```python
from build123d import *

# Parameters (mm, degrees)
SKETCH_1_R               = 6.325
EXTRUDE_1_DEPTH          = 15
SKETCH_2_W               = 20.7
SKETCH_2_H               = 20
EXTRUDE_2_DEPTH          = 5
SKETCH_3_W               = 5
SKETCH_3_H               = 20
EXTRUDE_3_DEPTH          = 10.2
SKETCH_4_R               = 1.7
CUT_EXTRUDE_1_DEPTH      = 21.932331452
CUT_EXTRUDE_1_DEPTH_BACK = 21.932331452
SKETCH_5_R               = 1.65
CUT_EXTRUDE_2_DEPTH      = 21.932331452
CUT_EXTRUDE_2_DEPTH_BACK = 21.932331452
SKETCH_6_R               = 1.75
EXTRUDE_4_DEPTH          = 5
CHAMFER_2_SIZE           = 1
CHAMFER_3_SIZE           = 1
CUT_EXTRUDE_3_DEPTH      = 33.153149146
CUT_EXTRUDE_3_DEPTH_BACK = 33.153149146
SKETCH_9_R               = 12.25
SKETCH_9_R_2             = 9.25
EXTRUDE_5_DEPTH          = 15
SKETCH_10_R              = 14.05
EXTRUDE_6_DEPTH          = 2
CUT_EXTRUDE_4_DEPTH      = 31.356342006
CUT_EXTRUDE_4_DEPTH_BACK = 31.356342006
CUT_EXTRUDE_5_REACH      = 44.837
SKETCH_12_W              = 4.440498429
SKETCH_12_H              = 7
SKETCH_12_W_2            = 5.469845286


with BuildPart() as part:
    # ｽｹｯﾁ1 → ﾎﾞｽ - 押し出し1 (new body)
    with BuildSketch(Plane.XY):
        Circle(SKETCH_1_R)
    extrude(amount=-EXTRUDE_1_DEPTH)

    # ｽｹｯﾁ2 → ﾎﾞｽ - 押し出し2 (add)
    with BuildSketch(Plane.XY):
        Rectangle(SKETCH_2_W, SKETCH_2_H)
    extrude(amount=EXTRUDE_2_DEPTH)

    # ｽｹｯﾁ3 → ﾎﾞｽ - 押し出し3 (add)
    with BuildSketch(Plane.XY.offset(5)):
        with Locations((7.85, 0)):
            Rectangle(SKETCH_3_W, SKETCH_3_H)
        with Locations((-7.85, 0)):
            Rectangle(SKETCH_3_W, SKETCH_3_H)
    extrude(amount=EXTRUDE_3_DEPTH)

    # ｽｹｯﾁ4 → ｶｯﾄ - 押し出し1 (cut, two sides)
    with BuildSketch(Plane(origin=(0, 0, 0), x_dir=(0, 0, -1), z_dir=(1, 0, 0))) as cut_extrude_1_sk:
        with Locations((-10.2, 5)):
            Circle(SKETCH_4_R)
        with Locations(Location((-10.2, -5, 0), (0, 0, 270))):
            Circle(SKETCH_4_R)
    extrude(amount=CUT_EXTRUDE_1_DEPTH, mode=Mode.SUBTRACT)
    extrude(cut_extrude_1_sk.sketch, amount=-CUT_EXTRUDE_1_DEPTH_BACK, mode=Mode.SUBTRACT)

    # ｽｹｯﾁ5 → ｶｯﾄ - 押し出し2 (cut, two sides)
    with BuildSketch(Plane(origin=(0, 0, 0), x_dir=(0, 0, -1), z_dir=(1, 0, 0))) as cut_extrude_2_sk:
        with Locations((7.5, 0)):
            Circle(SKETCH_5_R)
    extrude(amount=CUT_EXTRUDE_2_DEPTH, mode=Mode.SUBTRACT)
    extrude(cut_extrude_2_sk.sketch, amount=-CUT_EXTRUDE_2_DEPTH_BACK, mode=Mode.SUBTRACT)

    # ｽｹｯﾁ6 → ﾎﾞｽ - 押し出し4 (add)
    with BuildSketch(Plane.ZY.offset(10.35)):
        with BuildLine():
            Line((15.2, 10), (21.630535845, 3.285410753))
            ThreePointArc((21.630535845, 3.285410753), (22.95, 0), (21.630535845, -3.285410753))
            Line((21.630535845, -3.285410753), (15.2, -10))
            Line((15.2, -10), (15.2, 10))
        make_face()
        with Locations(Location((18.2, 0, 0), (0, 0, 270))):
            Circle(SKETCH_6_R, mode=Mode.SUBTRACT)
    extrude_4 = extrude(amount=-EXTRUDE_4_DEPTH)

    # ﾐﾗｰ1: ﾎﾞｽ - 押し出し4 across plane
    add(extrude_4.mirror(Plane(origin=(0, 0, 0), x_dir=(0, 0, 1), z_dir=(1, 0, 0))))

    # 面取り2
    chamfer_2_edges = [part.edges().sort_by_distance(p)[0] for p in [
        (10.35, -10, 7.6),
        (10.35, 10, 7.6),
        (-10.35, -6.642705377, 18.415267922),
        (-10.35, 0, 22.95),
        (-10.35, 6.642705377, 18.415267922),
        (-10.35, 10, 7.6),
        (-10.35, -10, 7.6),
        (10.35, -6.642705377, 18.415267922),
        (10.35, 0, 22.95),
        (10.35, 6.642705377, 18.415267922),
    ]]
    chamfer(chamfer_2_edges, length=CHAMFER_2_SIZE)

    # 面取り3
    chamfer_3_edges = [part.edges().sort_by_distance(p)[0] for p in [
        (-6.325, 0, -15),
    ]]
    chamfer(chamfer_3_edges, length=CHAMFER_3_SIZE)

    # ｽｹｯﾁ8 → ｶｯﾄ - 押し出し3 (cut, two sides)
    with BuildSketch(Plane(origin=(0, 10, 0), x_dir=(1, 0, 0), z_dir=(0, 1, 0))) as cut_extrude_3_sk:
        Polygon((-104.749244062, 0), (-16.325065883, 0), (21.444424523, 0), (109.868602701, 0), (109.868602701, 176.848356357), (-104.749244062, 176.848356357), align=None)
    extrude(amount=CUT_EXTRUDE_3_DEPTH, mode=Mode.SUBTRACT)
    extrude(cut_extrude_3_sk.sketch, amount=-CUT_EXTRUDE_3_DEPTH_BACK, mode=Mode.SUBTRACT)

    # ｽｹｯﾁ9 → ﾎﾞｽ - 押し出し5 (add)
    with BuildSketch(Plane(origin=(0, 0, 0), x_dir=(-1, 0, 0), z_dir=(0, 0, -1))):
        with Locations(Location((0, 0, 0), (0, 0, 212.338995303))):
            Circle(SKETCH_9_R)
        Circle(SKETCH_9_R_2, mode=Mode.SUBTRACT)
    extrude(amount=EXTRUDE_5_DEPTH)

    # ｽｹｯﾁ10 → ﾎﾞｽ - 押し出し6 (add)
    with BuildSketch(Plane.XY):
        Circle(SKETCH_10_R)
    extrude(amount=EXTRUDE_6_DEPTH)

    # ｽｹｯﾁ11 → ｶｯﾄ - 押し出し4 (cut, two sides)
    with BuildSketch(Plane(origin=(0, 0, 0), x_dir=(0, 0, -1), z_dir=(1, 0, 0))) as cut_extrude_4_sk:
        with BuildLine():
            Line((6.071058084, 0.825), (5.594744112, 0))
            Line((5.594744112, 0), (6.071058084, -0.825))
            ThreePointArc((6.071058084, -0.825), (9.15, 0), (6.071058084, 0.825))
        make_face()
    extrude(amount=CUT_EXTRUDE_4_DEPTH, mode=Mode.SUBTRACT)
    extrude(cut_extrude_4_sk.sketch, amount=-CUT_EXTRUDE_4_DEPTH_BACK, mode=Mode.SUBTRACT)

    # ｶｯﾄ - 押し出し5: up to this face of the body (flat: up to its plane)
    cut_extrude_5_end = Plane(part.part.faces().sort_by_distance((-10.685757389, 6.765438958, 0))[0])
    # ｽｹｯﾁ12 → ｶｯﾄ - 押し出し5 (cut, up to the picked face)
    with BuildSketch(Plane(origin=(0, 0, -15), x_dir=(-1, 0, 0), z_dir=(0, 0, -1)), mode=Mode.PRIVATE) as cut_extrude_5_sk1:
        with Locations((-13.959606096, 0)):
            Rectangle(SKETCH_12_W, SKETCH_12_H)
    cut_extrude_5_tool1 = split(extrude(cut_extrude_5_sk1.sketch, amount=-CUT_EXTRUDE_5_REACH, mode=Mode.PRIVATE), bisect_by=cut_extrude_5_end, keep=Keep.BOTH, mode=Mode.PRIVATE)
    # ｽｹｯﾁ12 → ｶｯﾄ - 押し出し5 (cut, up to the picked face)
    with BuildSketch(Plane(origin=(0, 0, -15), x_dir=(-1, 0, 0), z_dir=(0, 0, -1)), mode=Mode.PRIVATE) as cut_extrude_5_sk2:
        with Locations((14.474279525, 0)):
            Rectangle(SKETCH_12_W_2, SKETCH_12_H)
    cut_extrude_5_tool2 = split(extrude(cut_extrude_5_sk2.sketch, amount=-CUT_EXTRUDE_5_REACH, mode=Mode.PRIVATE), bisect_by=cut_extrude_5_end, keep=Keep.BOTH, mode=Mode.PRIVATE)
    add(cut_extrude_5_tool1.solids().sort_by(Axis((13.959606, 0, -15), (0, 0, 1)))[0], mode=Mode.SUBTRACT)
    add(cut_extrude_5_tool2.solids().sort_by(Axis((-14.47428, 0, -15), (0, 0, 1)))[0], mode=Mode.SUBTRACT)


solid = part.part
```
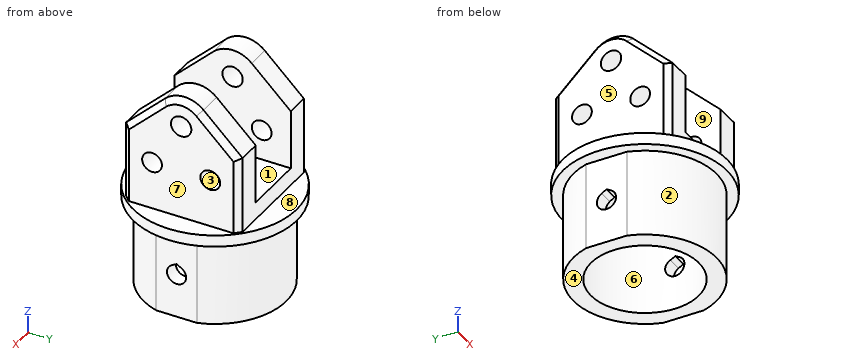
CAD build for the part. Positions are in the model's coordinates, mm. Face numbers are marked on the shaded views. A direction names the side the tool comes from. Round coordinates to 2 decimals unless told otherwise and drop trailing zeros. Order: outer loops, then holes, each group sorted by start corner. A loop starts at its lowest first (then second) coordinate and runs counter-clockwise, first axis right, second up.
Q1. Wall check: L1, parallel to Y at x = -9.1, z = 10.2; L2, parallel to Z at x = 10.8, y = 0; L3, parallel to X at y = -0.25, z = 11. Give the ranges that are in metal, low to high.
Q2. Drop flat-ended pins along their axis: pin 1 (5 mm diameter, centred on y = 0.5, z = -0.5, fed in from -X); pin 2 (5 mm diameter, centred on x = 3.5, z = -9.5, fed in from +Y); pin 3 (9 mm diameter, centred on y = 2, z = 10, fed in from -X); pin 4 (1.5 mm diameter, centred on x = -4.5, y = -3.5, fed in from +Z). Give the stop position or say it passes through.
Q3. Slice it at D-D (x = -6.25). Write the cut outline in (y, z), and give its area (3 significant figures).
Q4. Slice it at C-C (z = 18.2). Write the cut outline in (x, y).
Q5. Two-plate mould, pull along Z, no slides. Class the marked faces 1, 2, 3 and 4: pulls with the +Z half, pulls with the -Z half, needs draft (parallel to the pull), parting line crosses it, or undercut.
Q6. Slice it at B-B (y = -6.25). State how many separate pieces and enclosed holes the cut face has, and give its area (3 significant figures).
Q7. Slice it at A-A (z = -7.5). Write the cut outline in (x, y).
Q8. Which spindle directions (+Z, -Z, +X, -X, +Y, -Y) get a long thin tool onto all of the face, cutting with end or side? Do the marked faces 5, 6, 7, 8 and 9. Say none if no direction does.
Results below:
1. L1: y = -10 to -6.7, -3.3 to 3.3, 6.7 to 10
1. L2: z = -15 to -9.15, -5.59 to 2
1. L3: x = -10.35 to -5.35, 5.35 to 10.35
2. pin 1: stops at x = -14.05
2. pin 2: stops at y = 12.21
2. pin 3: stops at x = -10.35
2. pin 4: stops at z = 5
3. outline: (-12.58, 0) - (-10.54, 0) - (-10.54, -15) - (-6.82, -15) - (-6.82, 0) - (6.82, 0) - (6.82, -15) - (10.54, -15) - (10.54, 0) - (12.58, 0) - (12.58, 2) - (10, 2) - (10, 15.2) - (3.29, 21.63) arc R4.75 ccw to (-3.29, 21.63) - (-10, 15.2) - (-10, 2) - (-12.58, 2) - close; hole circle Ø3.4 at (-5, 10.2); hole circle Ø3.5 at (0, 18.2); hole circle Ø3.4 at (5, 10.2)
3. area: 489 mm2
4. outline: (-10.35, -5.42) - (-9.35, -6.87) - (-5.35, -6.87) - (-5.35, -1.75) - (-10.35, -1.75) - close; (-10.35, 1.75) - (-5.35, 1.75) - (-5.35, 6.87) - (-9.35, 6.87) - (-10.35, 5.42) - close; (5.35, -6.87) - (9.35, -6.87) - (10.35, -5.42) - (10.35, -1.75) - (5.35, -1.75) - close; (5.35, 1.75) - (10.35, 1.75) - (10.35, 5.42) - (9.35, 6.87) - (5.35, 6.87) - close
5. face 1: pulls with the +Z half
5. face 2: needs draft
5. face 3: undercut
5. face 4: pulls with the -Z half
6. separate pieces: 3
6. enclosed holes: 0
6. area: 337 mm2
7. outline: (-11.74, -3.5) arc R12.25 ccw to (11.74, -3.5) - (11.74, -1.65) - (9.1, -1.65) arc R9.25 cw to (-9.1, -1.65) - (-11.74, -1.65) - close; (-11.74, 1.65) - (-9.1, 1.65) arc R9.25 cw to (9.1, 1.65) - (11.74, 1.65) - (11.74, 3.5) arc R12.25 ccw to (-11.74, 3.5) - close
8. face 5: +Z, -X, +Y, -Y
8. face 6: -Z
8. face 7: +Z, +X, +Y, -Y
8. face 8: +Z
8. face 9: +Z, +Y, -Y
